Job drawing, mm, ordinate dimensions from the low corner. One solid piece. Coordinates: 2 decimals unless noted, no trailing zeros. Loops run counter-clockwise (first coordinate to the right, second up) from the corner with the lowest first, then second, coordinate; pieces in that order, holes last. Notation, with made-up numbers: M 54,15 L 70,15 A4 cw 70,20 Z; hole C 1.5,12.25 d6. An arc over 180 degrees is marked long. Answer as a JSON object with one key per item and string values. Group by question number.
1. Saw through at C-C on z = 146. Write the cut outline in (x, y), then the cut area to 3 significant figures.
2. Saw through at A-A on x = 30.5. Write the cut outline in (y, z), then the cut area to 3 significant figures.
3. Drop flat-ended pins along their axis: pin 1 Ø3.5 at (x, z) = (10, 52) entering from -Y; pin 2 Ø1 at (y, z) = (0.5, 116.5) entering from -X. Give the stop position or say it passes through.
4. Drill centre lines: L1, parallel to X at y = 1.3, z = 141.25; L2, parallel to Z at x = 115, y = 0.65; L3, parallel to X at y = 0.95, z = 172. Where is each one in solid material? Low to high.
5. Saw through at B-B on y = 0.8. Count the separate pieces of the cut face and the enclosed holes in it, then the cut area to 3 significant figures.
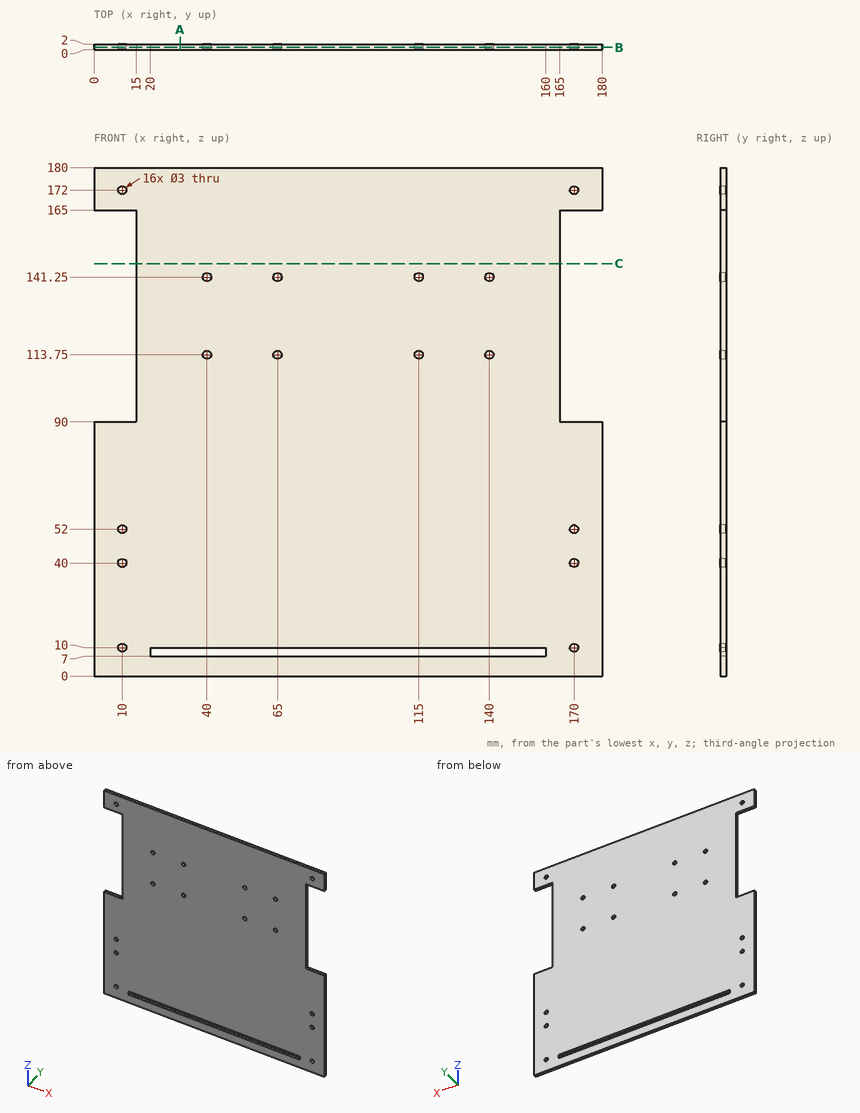
Outcome:
{
 "1": {"outline": "M 15,0 L 165,0 L 165,2 L 15,2 Z", "area": "300 mm²"},
 "2": {"outline": "M 0,0 L 2,0 L 2,7 L 0,7 Z; M 0,10 L 2,10 L 2,180 L 0,180 Z", "area": "354 mm²"},
 "3": {"pin 1": "stops at y = 0", "pin 2": "stops at x = 15"},
 "4": {"L1": "x = 15 to 38.5, 41.5 to 63.5, 66.5 to 113.5, 116.5 to 138.5, 141.5 to 165", "L2": "z = 0 to 7, 10 to 112.25, 115.25 to 139.75, 142.75 to 180", "L3": "x = 0 to 8.5, 11.5 to 168.5, 171.5 to 180"},
 "5": {"separate pieces": "1", "enclosed holes": "17", "area": "29,600 mm²"}
}
